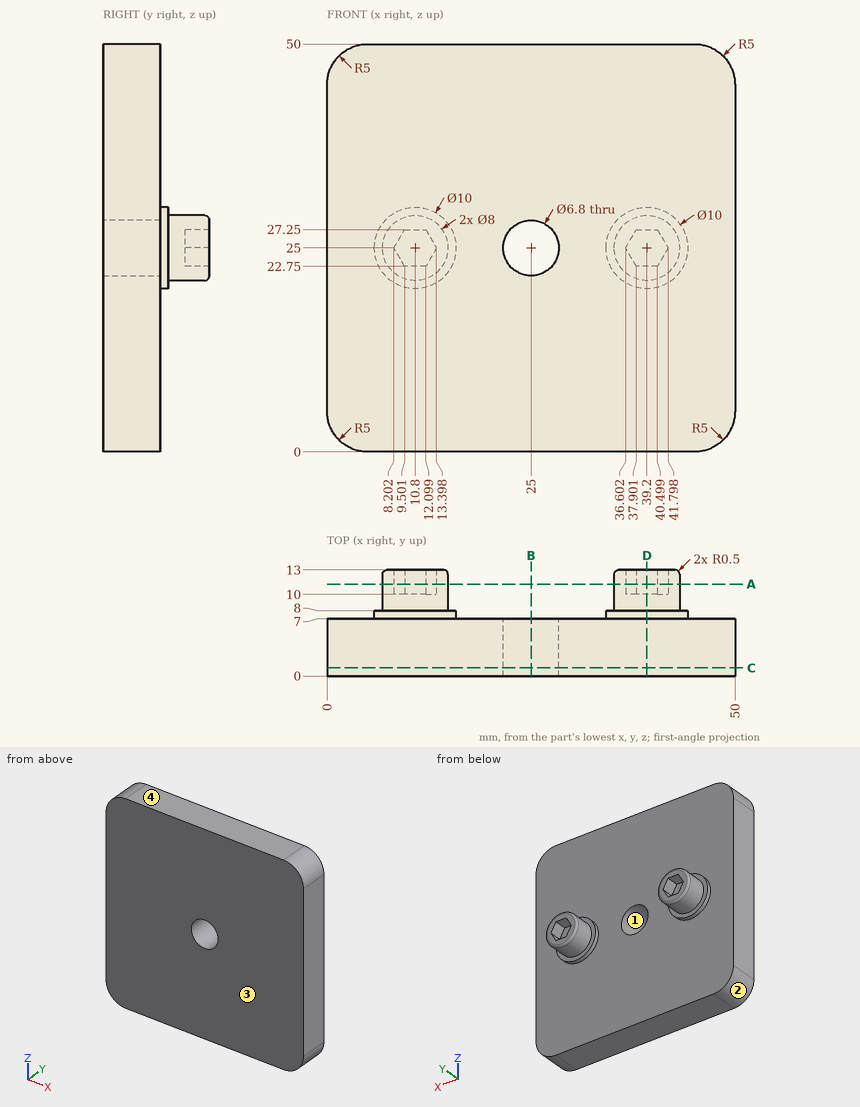
Can you work these out from the drawing? Everything is in mm from the part's minimum corner. Coordinates: 2 decimals unless noted, no trailing zeros. Loops run counter-clockwise (first coordinate to the right, second up) from the corner with the lowest first, then second, coordinate; pieces in that order, holes last.
1) Imagine slicing it at A-A (y = 11.25). List the corners of the cut face in (x, z) for me.
Reported:
outline: circle Ø8 at (10.8, 25); circle Ø8 at (39.2, 25); hole (8.2, 25) - (9.5, 22.75) - (12.1, 22.75) - (13.4, 25) - (12.1, 27.25) - (9.5, 27.25) - close; hole (36.6, 25) - (37.9, 22.75) - (40.5, 22.75) - (41.8, 25) - (40.5, 27.25) - (37.9, 27.25) - close
2) Imagine slicing it at D-D (x = 39.2). List the corners of the cut face in (y, z) for me, and give its area (3 significant figures).
Reported:
outline: (0, 0) - (7, 0) - (7, 20) - (8, 20) - (8, 21) - (12.5, 21) arc R0.5 ccw to (13, 21.5) - (13, 22.75) - (10, 22.75) - (10, 27.25) - (13, 27.25) - (13, 28.5) arc R0.5 ccw to (12.5, 29) - (8, 29) - (8, 30) - (7, 30) - (7, 50) - (0, 50) - close
area: 386 mm2
3) Imagine slicing it at B-B (x = 25). List the corners of the cut face in (y, z) for me, and give its area (3 significant figures).
Reported:
outline: (0, 0) - (7, 0) - (7, 21.6) - (0, 21.6) - close; (0, 28.4) - (7, 28.4) - (7, 50) - (0, 50) - close
area: 302 mm2
4) Will these pins go through, and if not, where does the flat tip stop? pin 1 Ø0.8 at (x, y) = (10.5, 11.5) entering from -Z; pin 2 Ø6 at (x, z) = (42.5, 41.5) entering from +Y; pin 3 Ø0.8 at (x, y) = (39, 11.5) entering from +Z.
Reported:
pin 1: stops at z = 21
pin 2: stops at y = 7
pin 3: stops at z = 29
5) Imagine slicing it at C-C (y = 1). List the corners of the cut face in (x, z) for me, and give its area (3 significant figures).
Reported:
outline: (0, 5) arc R5 ccw to (5, 0) - (45, 0) arc R5 ccw to (50, 5) - (50, 45) arc R5 ccw to (45, 50) - (5, 50) arc R5 ccw to (0, 45) - close; hole circle Ø6.8 at (25, 25)
area: 2,440 mm2
6) Thinking about a two-plate mould opening in Z: for the marked faces 1, 2, 3 and 4, which applies, released by +Z, released by -Z, zero draft, split by the parting line, or undercut?
Reported:
face 1: undercut
face 2: released by -Z
face 3: zero draft
face 4: released by +Z
7) Please list where these lines run through material, in increasing order: line 1 along X through (y, z) = (4.75, 25); line 2 along Y through (x, z) = (33.5, 20.5); line 3 along X through (y, z) = (7.75, 26.5).
Reported:
line 1: x = 0 to 21.6, 28.4 to 50
line 2: y = 0 to 7
line 3: x = 6.03 to 15.57, 34.43 to 43.97
